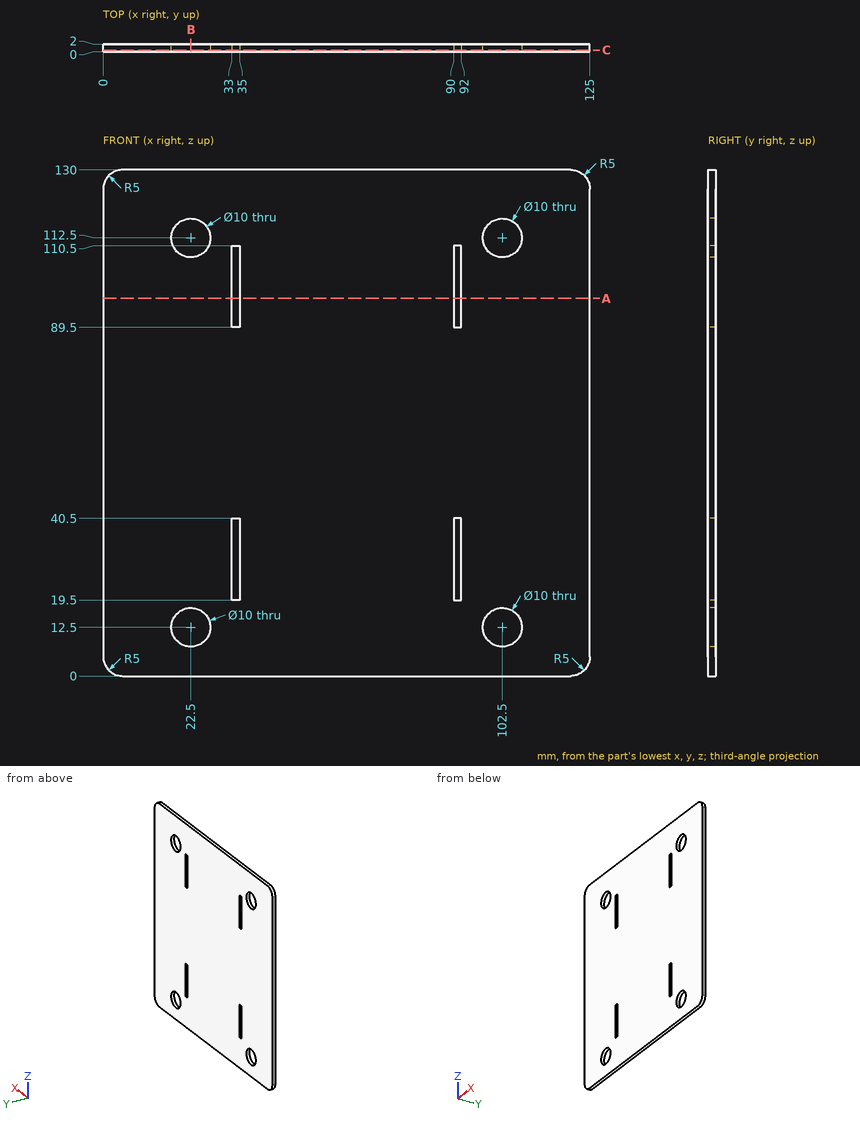
Answer from the drawing. Dimensions are ordinates in mm from the lowest x, y and z of the part. Coordinates: 2 decimals unless noted, no trailing zeros. Write each loop counter-clockwise with the first axis right and the second up, starting at its lowest first coordinate (ties: lowest second). Pieces come first, ordered by that corner, then holes. Notation, with made-up numbers: (7, 28) - (17, 28) arc R25 ccw to (17, 63) - close; hole circle Ø4 at (58, 67.25). An arc over 180 degrees is marked (long way). One line per question, with ' | ' between items.
Q1. Consider L1, parallel to Z at x = 22.5, y = 0.75; L2, parallel to X at y = 0.7, z = 106.5; L3, parallel to Z at x = 101, y = 1.6. Determine where each line is inside the solid, lowest interval first. Write a range as [from, to].
Result set:
L1: [0, 7.5], [17.5, 107.5], [117.5, 130] | L2: [0, 33], [35, 90], [92, 125] | L3: [0, 7.73], [17.27, 107.73], [117.27, 130]
Q2. Find section B-B, the plane x = 22.5. Write down the section's boundary in (y, z), plus the area to 3 significant figures.
Result set:
outline: (0, 0) - (2, 0) - (2, 7.5) - (0, 7.5) - close; (0, 17.5) - (2, 17.5) - (2, 107.5) - (0, 107.5) - close; (0, 117.5) - (2, 117.5) - (2, 130) - (0, 130) - close | area: 220 mm^2
Q3. Find section A-A, the plane z = 97. Write down the section's boundary in (x, y), plus the area to 3 significant figures.
Result set:
outline: (0, 0) - (33, 0) - (33, 2) - (0, 2) - close; (35, 0) - (90, 0) - (90, 2) - (35, 2) - close; (92, 0) - (125, 0) - (125, 2) - (92, 2) - close | area: 242 mm^2
Q4. This flat-tipped pin is pushed along its axis until it touches: P1, Ø1, axis at x = 91, z = 101, coming from the +Y side. Where does it stop, or does it pass through?
Result set:
P1: through
Q5. Find section C-C, the plane y = 0.45. State how many separate pieces and enclosed holes the cut face has, plus the area to 3 significant figures.
Result set:
separate pieces: 1 | enclosed holes: 8 | area: 15,700 mm^2
